```python
from build123d import *

# Parameters (mm, degrees)
SKETCH1_R           = 1.75
SKETCH1_R_2         = 1.25
BOSS_EXTRUDE1_DEPTH = 5


with BuildPart() as part:
    # Sketch1 → Boss-Extrude1 (new body)
    with BuildSketch(Plane.XY):
        with BuildLine():
            Line((274.735652315, 354.190888595), (274.735652315, 378.690888595))
            ThreePointArc((274.735652315, 378.690888595), (274.542108821, 380.137097205), (273.975099827, 381.481522444))
            Line((273.975099827, 381.481522444), (258.753460649, 407.333054329))
            ThreePointArc((258.753460649, 407.333054329), (251.662864877, 409.514553006), (248.849842147, 402.649978145))
            Line((248.849842147, 402.649978145), (250.029730466, 400.750917928))
            Line((250.029730466, 400.750917928), (263.735652315, 378.690888595))
            Line((263.735652315, 378.690888595), (263.735652315, 348.690888595))
            ThreePointArc((263.735652315, 348.690888595), (265.346565018, 344.801801299), (269.235652315, 343.190888595))
            Line((269.235652315, 343.190888595), (279.235652315, 343.190888595))
            Line((279.235652315, 343.190888595), (279.235652315, 354.190888595))
            Line((279.235652315, 354.190888595), (274.735652315, 354.190888595))
        make_face()
        with Locations((269.235652315, 348.690888595)):
            Circle(SKETCH1_R, mode=Mode.SUBTRACT)
        with Locations((254.014013137, 404.542420479)):
            Circle(SKETCH1_R_2, mode=Mode.SUBTRACT)
        with Locations((269.235652315, 378.690888595)):
            Circle(SKETCH1_R_2, mode=Mode.SUBTRACT)
    extrude(amount=BOSS_EXTRUDE1_DEPTH)


solid = part.part
```
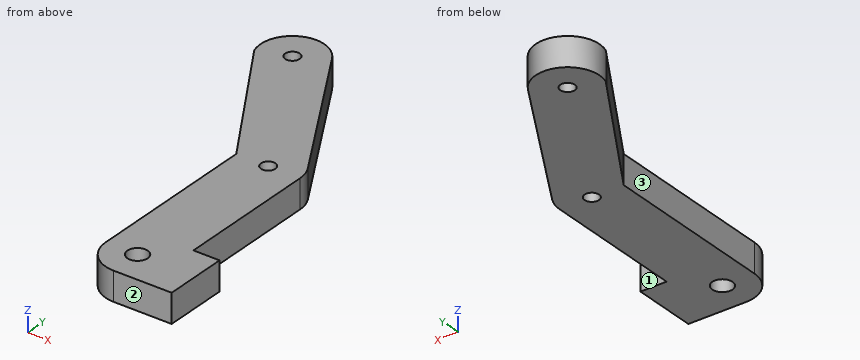
Build history of the part. All positions in model axes, mm. Face numbers are marked on the shaded views. A direction names the side the tool comes from. Round coordinates to 2 decimals unless told otherwise and drop trailing zeros. Write each loop counter-clockwise with the first axis right and the second up, starting at its lowest first coordinate (ties: lowest second). Pieces come first, ordered by that corner, then holes. Notation, with made-up numbers: (-24, 65) -> (20, 65) arc R32 cw to (20, 95) -> close; hole circle Ø1 at (47.5, -1). An arc over 180 degrees is marked (long way). Put each result on its own line as item: value.
Item 1: Slice it at A-A, the plane z = 2.9. Give the cut face in (x, y).
Here are the results:
outline: (248.85, 402.65) -> (263.74, 378.69) -> (263.74, 348.69) arc R5.5 ccw to (269.24, 343.19) -> (279.24, 343.19) -> (279.24, 354.19) -> (274.74, 354.19) -> (274.74, 378.69) arc R5.5 ccw to (273.98, 381.48) -> (258.75, 407.33) arc R5.5 ccw to start; hole circle Ø2.5 at (254.01, 404.54); hole circle Ø3.5 at (269.24, 348.69); hole circle Ø2.5 at (269.24, 378.69)
Item 2: Slice it at B-B, the plane y = 355.5. Give the cut face in (x, z), plus the area to 3 significant figures.
Here are the results:
outline: (263.74, 0) -> (274.74, 0) -> (274.74, 5) -> (263.74, 5) -> close
area: 55.0 mm^2
Item 3: Slice it at C-C, the plane x = 260.5. Give the cut face in (y, z), plus the area to 3 significant figures.
Here are the results:
outline: (383.9, 0) -> (404.37, 0) -> (404.37, 5) -> (383.9, 5) -> close
area: 102 mm^2
Item 4: Flat gauge pin, fed straight in: P1, Ø1.5, axis at y = 365, z = 2, coming from the +X side. Where does the tip first touch, or does it go through?
Here are the results:
P1: stops at x = 274.74
Item 5: Wall check: probe 1 along Y at (x, z) = (275.5, 1.8); probe 2 along X at (y, z) = (356.5, 0.3); probe 3 along X at (y, z) = (350, 2.8). Give the ranges that are in metal, low to high. Write a range as from..to.
Here are the results:
probe 1: y = 343.19..354.19
probe 2: x = 263.74..274.74
probe 3: x = 263.74..268.07, 270.4..279.24
Item 6: Tool access for the marked faces 1, 2 and 3: list every direction of +Z, -Z, +X, -X, +Y, -Y with a clear straight run to the whole face (end or side of a thin tool).
Here are the results:
face 1: +Z, -Z, +X, +Y
face 2: +Z, -Z, +X, -X, -Y
face 3: +Z, -Z, -X, -Y
